For this review, take the finished solid that the model builds, in its own axes (mm). Face numbers are marked on the shaded views. Round coordinates to 2 decimals unless told otherwise and drop trailing zeros. Write each loop counter-clockwise with the first axis right and the second up, starting at its lowest first coordinate (ties: lowest second). Pieces come first, ordered by that corner, then holes. Notation, with made-up numbers: M 64.25,85.25 L 121.25,85.25 A16 ccw 121.25,104.25 Z; hole C 87.25,52 d4. An arc over 180 degrees is marked long. Use one line per item in the form item = value. Start each with the question number.
Item 1: Add section D-D (z = 14.25). State the section outline as (x, y) points.
Item 2: Draft analysis for pull direction Y (two halves, no side actions). For the marked faces 1, 2 and 3, state which applies: released by +Y, released by -Y, zero draft, split by the parting line, or undercut.
Item 3: Add section B-B (z = 0). State the section outline as (x, y) points.
Item 4: For P1, Ø0.6, axis at x = -12.5, y = 23, coming from the +Z side; P2, Ø12, axis at y = 5.5, z = -6, coming from the -X side; P3, Ø1, axis at x = -11.5, y = 1, coming from the -Z side, all flat-tipped, find the tip position at first contact; note any pin that passes through.
Item 5: Add section C-C (x = -11). State the section outline as (y, z) points.
Item 6: For line 1 (X direction, y = 9.5, z = 16); line 2 (Y direction, x = -6.5, z = 10.25); line 3 (Z direction, x = 1.5, y = 7.25), list the stretches that pass through material, from the lowest coordinate up. Write a range as [from, to].
Item 7: Add section A-A (y = 9). State the section outline as (x, z) points.
from build123d import *

# Parameters (mm, degrees)
SKETCH2_W           = 10
SKETCH2_H           = 27
BOSS_EXTRUDE1_DEPTH = 24
SKETCH3_R           = 6.75
CUT_EXTRUDE1_DEPTH  = 10
SKETCH6_W           = 8
SKETCH6_H           = 2
BOSS_EXTRUDE2_DEPTH = 32
FILLET1_RADIUS      = 4
FILLET1_LENGTH      = 2
SKETCH8_R           = 1.5
CUT_EXTRUDE2_DEPTH  = 2
SKETCH10_W          = 8
SKETCH10_H          = 2
BOSS_EXTRUDE3_DEPTH = 22
FILLET2_RADIUS      = 4
FILLET2_LENGTH      = 2
SKETCH11_R          = 1.5
CUT_EXTRUDE4_DEPTH  = 2


with BuildPart() as part:
    # Sketch2 → Boss-Extrude1 (new body)
    with BuildSketch(Plane(origin=(0, 0, 0), x_dir=(1, 0, 0), z_dir=(0, 1, 0))):
        with Locations((0, -4.5)):
            Rectangle(SKETCH2_W, SKETCH2_H)
    extrude(amount=BOSS_EXTRUDE1_DEPTH)

    # Sketch3 → Cut-Extrude1 (cut)
    with BuildSketch(Plane(origin=(5, 0, 0), x_dir=(0, 0, -1), z_dir=(1, 0, 0))):
        with Locations((0, 9)):
            Circle(SKETCH3_R)
    extrude(amount=-CUT_EXTRUDE1_DEPTH, mode=Mode.SUBTRACT)

    # Sketch6 → Boss-Extrude2 (add)
    with BuildSketch(Plane(origin=(5, 0, 0), x_dir=(0, 0, -1), z_dir=(1, 0, 0))):
        with Locations((0, 23)):
            Rectangle(SKETCH6_W, SKETCH6_H)
    extrude(amount=-BOSS_EXTRUDE2_DEPTH)

    # Fillet1: full round fillet: the end face becomes a half cylinder, R = half its width
    fillet1_face = Plane((-27, 23, 0), x_dir=(0, 1, 0), z_dir=(-1, 0, 0))  # on the end face: x along it, z out of the body
    fillet1_slab = fillet1_face.offset(-FILLET1_RADIUS / 2) * Box(FILLET1_LENGTH, 2 * FILLET1_RADIUS, FILLET1_RADIUS, mode=Mode.PRIVATE)  # the body's end, R deep
    fillet1_round = Plane((-23, 23, 0), x_dir=(-1, 0, 0), z_dir=(0, 1, 0)) * Cylinder(FILLET1_RADIUS, FILLET1_LENGTH, mode=Mode.PRIVATE)  # its axis R under the face
    add(fillet1_slab - fillet1_round, mode=Mode.SUBTRACT)

    # Sketch8 → Cut-Extrude2 (cut)
    with BuildSketch(Plane(origin=(0, 24, 0), x_dir=(1, 0, 0), z_dir=(0, 1, 0))):
        with Locations(Location((-23, 0, 0), (0, 0, 270))):
            Circle(SKETCH8_R)
    extrude(amount=-CUT_EXTRUDE2_DEPTH, mode=Mode.SUBTRACT)

    # Sketch10 → Boss-Extrude3 (add)
    with BuildSketch(Plane.ZY.offset(5)):
        with Locations((14, 1)):
            Rectangle(SKETCH10_W, SKETCH10_H)
    extrude(amount=BOSS_EXTRUDE3_DEPTH)

    # Fillet2: full round fillet: the end face becomes a half cylinder, R = half its width
    fillet2_face = Plane((-27, 1, 14), x_dir=(0, 1, 0), z_dir=(-1, 0, 0))  # on the end face: x along it, z out of the body
    fillet2_slab = fillet2_face.offset(-FILLET2_RADIUS / 2) * Box(FILLET2_LENGTH, 2 * FILLET2_RADIUS, FILLET2_RADIUS, mode=Mode.PRIVATE)  # the body's end, R deep
    fillet2_round = Plane((-23, 1, 14), x_dir=(-1, 0, 0), z_dir=(0, 1, 0)) * Cylinder(FILLET2_RADIUS, FILLET2_LENGTH, mode=Mode.PRIVATE)  # its axis R under the face
    add(fillet2_slab - fillet2_round, mode=Mode.SUBTRACT)

    # Sketch11 → Cut-Extrude4 (cut)
    with BuildSketch(Plane(origin=(0, 2, 0), x_dir=(1, 0, 0), z_dir=(0, 1, 0))):
        with Locations(Location((-23, -14, 0), (0, 0, 270))):
            Circle(SKETCH11_R)
    extrude(amount=-CUT_EXTRUDE4_DEPTH, mode=Mode.SUBTRACT)


solid = part.part
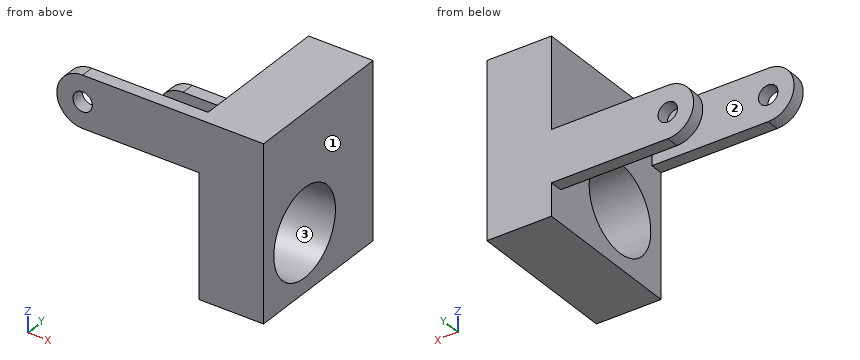
Calculated:
q1.outline = M -26.99,0 L -24.48,0 L -24.48,2 L -26.99,2 Z; M -21.52,0 L 5,0 L 5,24 L -5,24 L -5,2 L -21.52,2 Z
q2.face_1 = zero draft
q2.face_2 = released by +Y
q2.face_3 = undercut
q3.outline = M -27,22 L -24.5,22 L -24.5,24 L -27,24 Z; M -21.5,22 L -5,22 L -5,15.75 L 5,15.75 L 5,24 L -21.5,24 Z; M -5,0 L 5,0 L 5,2.25 L -5,2.25 Z
q4.P1 = 4
q4.P2 = -5
q4.P3 = 10
q5.outline = M 0,10 L 2,10 L 2,18 L 0,18 Z; M 22,-4 L 24,-4 L 24,4 L 22,4 Z
q6.line_1 = [-5, 5]
q6.line_2 = [0, 2]
q6.line_3 = [-9, -6.52], [6.52, 18]
q7.outline = M -5,-9 L 5,-9 L 5,-6.75 L -5,-6.75 Z; M -5,6.75 L 5,6.75 L 5,18 L -5,18 Z
